from build123d import *

# Parameters (mm, degrees)
SKETCH1_R           = 5
BOSS_EXTRUDE2_DEPTH = 3


with BuildPart() as part:
    # Sketch1 → Boss-Extrude2 (new body)
    # profile 1 of 6: a face of its own
    with BuildSketch(Plane.XY):
        with BuildLine():
            ThreePointArc((22.5, 0), (15.909902577, 15.909902577), (0, 22.5))
            Line((0, 22.5), (-22.5, 0))
            Line((-22.5, 0), (-22.124973736, -4.090909091))
            ThreePointArc((-22.124973736, -4.090909091), (2.054031517, -22.406047276), (22.5, 0))
        make_face()
        Circle(SKETCH1_R, mode=Mode.SUBTRACT)
    # profile 2 of 6: a face of its own
    with BuildSketch(Plane.XY):
        with BuildLine():
            ThreePointArc((-22.5, 0), (-15.909902577, 15.909902577), (0, 22.5))
            Line((0, 22.5), (-22.5, 22.5))
            Line((-22.5, 22.5), (-22.5, 0))
        make_face()
    # profile 3 of 6: a face of its own
    with BuildSketch(Plane.XY):
        with BuildLine():
            Line((-22.5, 0), (0, 22.5))
            ThreePointArc((0, 22.5), (-15.909902577, 15.909902577), (-22.5, 0))
        make_face()
    # profile 4 of 6: a face of its own
    with BuildSketch(Plane.XY):
        Polygon((-27.041634566, 0), (-22.5, 0), (-22.5, 22.5), (-79.5, 22.5), (-79.5, 0), align=None)
    # profile 5 of 6: a face of its own
    with BuildSketch(Plane.XY):
        with BuildLine():
            ThreePointArc((-22.124973736, -4.090909091), (-22.406047276, -2.054031517), (-22.5, 0))
            Line((-22.5, 0), (-27.041634566, 0))
            ThreePointArc((-27.041634566, 0), (-23.843623821, -1.156469426), (-22.124973736, -4.090909091))
        make_face()
    # profile 6 of 6: a face of its own
    with BuildSketch(Plane.XY):
        with BuildLine():
            Line((-22.124973736, -4.090909091), (-22.5, 0))
            ThreePointArc((-22.5, 0), (-22.406047276, -2.054031517), (-22.124973736, -4.090909091))
        make_face()
    extrude(amount=BOSS_EXTRUDE2_DEPTH)


solid = part.part
Read the model definition and answer for the solid it produces. Units are mm, in the model's axes. A direction names the side the tool comes from. Round coordinates to 2 decimals unless told otherwise and drop trailing zeros. Order: outer loops, then holes, each group sorted by start corner. A loop starts at its lowest first (then second) coordinate and runs counter-clockwise, first axis right, second up. Notation, with made-up numbers: (-1, 4.5) - (55, 4.5) arc R18 ccw to (55, 8.5) - close; hole circle Ø7 at (86.25, -10). An arc over 180 degrees is marked (long way). Use one line per item in the form item = value. Start each with the question number.
(1) A flat-ended cylindrical pin translates along its axis: pin 1 Ø1.5 at (x, z) = (-64, 1) entering from -Y. Find the tip coordinate at first contact, or state that the pin passes through.
(2) For faces 1 (the face through (-79.5, 11, 1)), 2 (the face through (-54, 0, 1)), determine the directions among +Z, -Z, +X, -X, +Y, -Y from which every point of the face is accessible in a straight line to the end or side of a thin tool.
(3) Find the intervals of material crossed by line 1 along Y through (x, z) = (0, 1.75); line 2 along X through (y, z) = (-3.5, 0.55); line 3 along Y through (x, z) = (-31, 0.7), in increasing order. Write a range as from..to.
(4) The part is cut by section A-A (z = 1.2). Give the vertices of the cut face in (x, y), then the cut area to 3 significant figures.
(5) The part is cut by section B-B (x = 2). Give the vertices of the cut face in (y, z).
(6) The part is cut by section C-C (x = -34.5). Give the vertices of the cut face in (y, z).
(7) The part is cut by section D-D (y = 16). Give the vertices of the cut face in (x, z), then the cut area to 3 significant figures.
(8) Determine the mould class of faces 3 (the face through (-23.881, -1.126, 1.479)), 4 (the face through (-1.08, -4.88, 1.48)), 5 (the face through (-29, 5, 3)), 6 (the face through (-39, 22.5, 1)) for opening direction Y: +Y half, -Y half, draft (parallel to the pull), parting line (faces both ways), or undercut.
Checked values:
q1.pin_1 = 0
q2.face_1 = +Z, -Z, -X, +Y, -Y
q2.face_2 = +Z, -Z, -X, -Y
q3.line_1 = -22.5..-5, 5..22.5
q3.line_2 = -22.27..-3.57, 3.57..22.23
q3.line_3 = 0..22.5
q4.outline = (-79.5, 0) - (-27.04, 0) arc R5 cw to (-22.12, -4.09) arc R22.5 ccw (long way) to (0, 22.5) - (-79.5, 22.5) - close; hole circle Ø10 at (0, 0)
q4.area = 2,910 mm^2
q5.outline = (-22.41, 0) - (-4.58, 0) - (-4.58, 3) - (-22.41, 3) - close; (4.58, 0) - (22.41, 0) - (22.41, 3) - (4.58, 3) - close
q6.outline = (0, 0) - (22.5, 0) - (22.5, 3) - (0, 3) - close
q7.outline = (-79.5, 0) - (15.82, 0) - (15.82, 3) - (-79.5, 3) - close
q7.area = 286 mm^2
q8.face_3 = -Y half
q8.face_4 = undercut
q8.face_5 = draft
q8.face_6 = +Y half
